The listing builds one solid part. Answer for the finished solid, in the listing's coordinates (mm). A direction names the side the tool comes from. Give positions to 0.01 mm unless a question says otherwise; leave off trailing zeros. Order: outer loops, then holes, each group sorted by start corner. A loop starts at its lowest first (then second) coordinate and runs counter-clockwise, first axis right, second up. Notation, with made-up numbers: (73, -2.5) - (83, -2.5) arc R35 ccw to (83, 35.5) - close; hole circle Ø4 at (58, -35.75). An arc over 180 degrees is marked (long way). Answer as CSV lines item,"result". Start each with the question number.
1. Section D-D on z = 39 is taken. Give the vertices of the cut face in (x, y), and give its area (3 significant figures).
2. Section C-C on z = 53.5 is taken. Give the vertices of the cut face in (x, y).
3. Flat-ended cylindrical pins translate along their axes: pin 1 (5 mm diameter, centred on y = 20, z = 46, fed in from -X); pin 2 (9 mm diameter, centred on y = 13, z = 33, fed in from -X); pin 3 (3 mm diameter, centred on x = 70, z = 28, fed in from +Y). Find the tip coordinate at first contact, or state that the pin passes through.
4. Section B-B on y = 19 is taken. Give the vertices of the cut face in (x, z).
5. Consider line 1 along Z through (x, y) = (42.5, 23); line 2 along Z through (x, y) = (10.5, 6); line 3 along X through (y, z) = (16.5, 11). Determine where each line is inside the solid, lowest interval first. Write a range as [from, to].
6. Section A-A on x = 47 is taken. Give the vertices of the cut face in (y, z).
7. Which of the six approach directions +Z, -Z, +X, -X, +Y, -Y give full straight-line access (tool end or side, diameter ignored) to faces 5 (the flat face through (8, 14, 50)), 6 (the flat face through (70.73, 3.31, 28.59))?
8. Determine the mould class of faces 1 (the flat face through (43, 20, 44)), 2 (the flat face through (8, 14, 8)), 3 (the flat face through (39, 0, 9)), 4 (the flat face through (39, 25, 0)) for opening direction Z: +Z half, -Z half, draft (parallel to the pull), parting line (faces both ways), or undercut.
from build123d import *

# Parameters (mm, degrees)
SKETCH1_R           = 7.5
BOSS_EXTRUDE1_DEPTH = 58
SKETCH2_W           = 16
SKETCH2_H           = 42
CUT_EXTRUDE1_DEPTH  = 107.60206377
SKETCH3_W           = 38
SKETCH3_H           = 30
CUT_EXTRUDE2_DEPTH  = 107.60206377
CUT_EXTRUDE3_DEPTH  = 107.60206377


with BuildPart() as part:
    # Sketch1 → Boss-Extrude1 (new body)
    with BuildSketch(Plane.XY):
        with BuildLine():
            Line((0, 0), (65, 0))
            Line((65, 0), (80, 8.660254038))
            Line((80, 8.660254038), (80, 31.339745962))
            Line((80, 31.339745962), (65, 40))
            Line((65, 40), (36.66060556, 40))
            ThreePointArc((36.66060556, 40), (16.66060556, 35.82575695), (0, 24))
            Line((0, 24), (0, 0))
        make_face()
        with Locations(Location((34, 19, 0), (0, 0, 180))):
            Circle(SKETCH1_R, mode=Mode.SUBTRACT)
    extrude(amount=BOSS_EXTRUDE1_DEPTH)

    # Sketch2 → Cut-Extrude1 (cut, through all)
    with BuildSketch(Plane(origin=(0, 0, 0), x_dir=(1, 0, 0), z_dir=(0, 1, 0))):
        with Locations((8, -29)):
            Rectangle(SKETCH2_W, SKETCH2_H)
    extrude(amount=CUT_EXTRUDE1_DEPTH, mode=Mode.SUBTRACT)

    # Sketch3 → Cut-Extrude2 (cut, through all)
    with BuildSketch(Plane(origin=(0, 0, 0), x_dir=(1, 0, 0), z_dir=(0, 1, 0))):
        with Locations((35, -29)):
            Rectangle(SKETCH3_W, SKETCH3_H)
    extrude(amount=CUT_EXTRUDE2_DEPTH, mode=Mode.SUBTRACT)

    # Sketch4 → Cut-Extrude3 (cut, through all)
    with BuildSketch(Plane(origin=(0, 0, 0), x_dir=(1, 0, 0), z_dir=(0, 1, 0))):
        Polygon((65, 0), (80, -15), (80, 0), align=None)
        Polygon((65, -58), (80, -43), (80, -58), align=None)
    extrude(amount=CUT_EXTRUDE3_DEPTH, mode=Mode.SUBTRACT)


solid = part.part
Checks:
1,outline,"(54, 0) - (65, 0) - (80, 8.66) - (80, 31.34) - (65, 40) - (54, 40) - close"
1,area,"910 mm²"
2,outline,"(0, 0) - (65, 0) - (69.5, 2.6) - (69.5, 37.4) - (65, 40) - (36.66, 40) arc R50 ccw to (0, 24) - close; hole circle Ø15 at (34, 19)"
3,pin 1,"stops at x = 16"
3,pin 2,"stops at x = 54"
3,pin 3,"stops at y = 37.98"
4,outline,"(0, 0) - (26.5, 0) - (26.5, 14) - (16, 14) - (16, 8) - (0, 8) - close; (0, 50) - (16, 50) - (16, 44) - (26.5, 44) - (26.5, 58) - (0, 58) - close; (41.5, 0) - (65, 0) - (80, 15) - (80, 43) - (65, 58) - (41.5, 58) - (41.5, 44) - (54, 44) - (54, 14) - (41.5, 14) - close"
5,line 1,"z = [0, 14], [44, 58]"
5,line 2,"z = [0, 8], [50, 58]"
5,line 3,"x = [16, 26.93], [41.07, 76]"
6,outline,"(0, 0) - (40, 0) - (40, 14) - (0, 14) - close; (0, 44) - (40, 44) - (40, 58) - (0, 58) - close"
7,face 5,"-X, +Y, -Y"
7,face 6,"+Z, -Z, +X, -Y"
8,face 1,"undercut"
8,face 2,"undercut"
8,face 3,"draft"
8,face 4,"-Z half"
